Verification items for this drawing (mm, ordinates from the low corner). Round coordinates to 2 decimals unless told otherwise and drop trailing zeros. Loops run counter-clockwise (first coordinate to the right, second up) from the corner with the lowest first, then second, coordinate; pieces in that order, holes last. Notation, with made-up numbers: (8, 29) - (33, 29) arc R21 cw to (33, 62) - close; hole circle Ø1 at (80, 14.5). An arc over 180 degrees is marked (long way). Use a Markdown table: item, result. Add a question column.
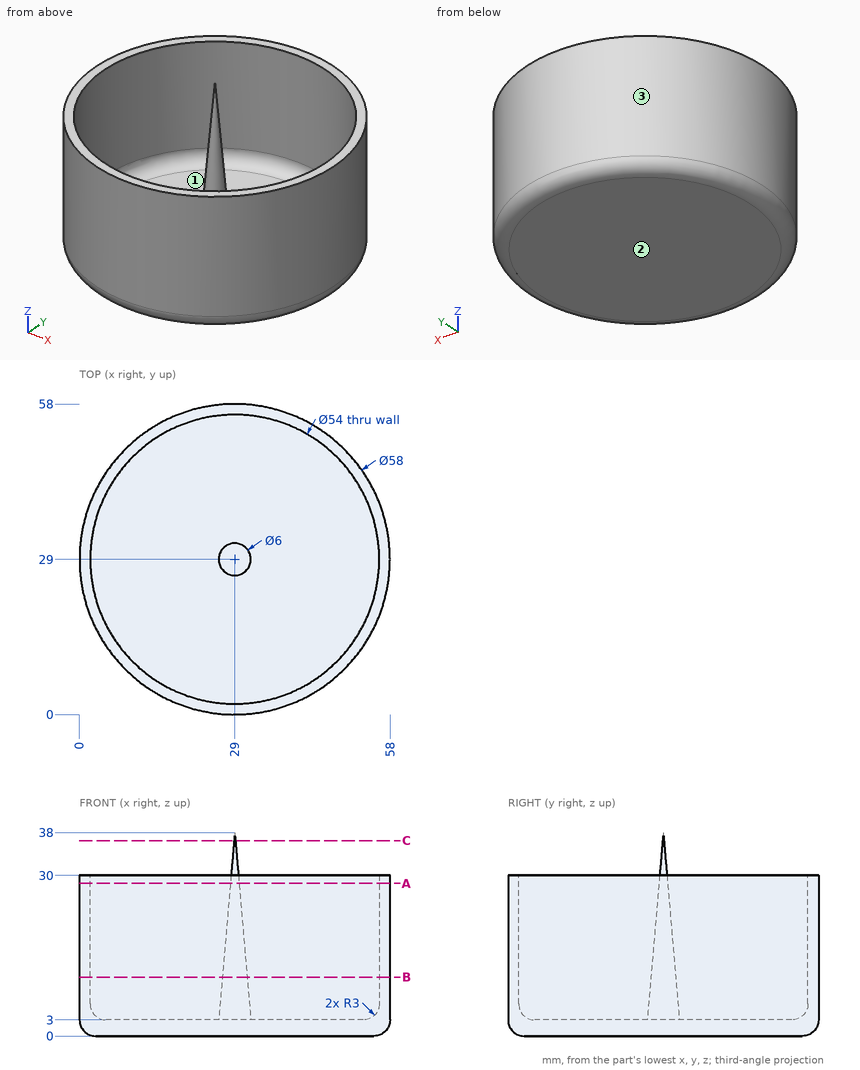
Q1. Section check C-C on z = 36.5. Record the cut outline in (x, y).
Q2. Release check for a two-part mould opening along X. For the marked faces 1, 2 and 3 record: +X half, -X half, draft (parallel to the pull), parting line (faces both ways), or undercut.
Q3. Thickness scan on line 1 along Y through (x, z) = (28, 20.5); line 2 along Y through (x, z) = (29, 15.25); line 3 along X through (y, z) = (16, 13). Record the ranges inside material, lowest first.
Q4. Section check A-A on z = 28.5. Record the cut outline in (x, y), plus the area to 3 significant figures.
Q5. Go/stop test with flat-tipped pins: pin 1 Ø3 at (x, z) = (21.5, 28.5) entering from -Y; pin 2 Ø1 at (x, y) = (10.5, 50.5) entering from +Z; pin 3 Ø4 at (x, z) = (33.5, 20) entering from -Y. Record where each tip stops, or that it passes through.
Q6. Section check B-B on z = 11. Record the cut outline in (x, y).
Determined:
| question | item | result |
|---|---|---|
| 1 | outline | circle Ø0.26 at (29, 29) |
| 2 | face 1 | undercut |
| 2 | face 2 | draft |
| 2 | face 3 | parting line |
| 3 | line 1 | y = 0.02 to 2.02, 27.88 to 30.12, 55.98 to 57.98 |
| 3 | line 2 | y = 0 to 2, 27.05 to 30.95, 56 to 58 |
| 3 | line 3 | x = 3.08 to 5.34, 52.66 to 54.92 |
| 4 | outline | circle Ø58 at (29, 29); circle Ø1.63 at (29, 29); hole circle Ø54 at (29, 29) |
| 4 | area | 354 mm² |
| 5 | pin 1 | stops at y = 0.63 |
| 5 | pin 2 | stops at z = 30 |
| 5 | pin 3 | stops at y = 0.11 |
| 6 | outline | circle Ø58 at (29, 29); circle Ø4.63 at (29, 29); hole circle Ø54 at (29, 29) |
